```python
from build123d import *

# Parameters (mm, degrees)
ESQUISSE1_W             = 61
ESQUISSE1_H             = 78
BOSS_EXTRU_1_DEPTH      = 2
ESQUISSE2_W             = 61
ESQUISSE2_H             = 78
ESQUISSE2_W_2           = 57
ESQUISSE2_H_2           = 74
BOSS_EXTRU_2_DEPTH      = 7
ESQUISSE3_W             = 59
ESQUISSE3_H             = 76
ESQUISSE3_W_2           = 57
ESQUISSE3_H_2           = 74
BOSS_EXTRU_3_DEPTH      = 4
ESQUISSE4_R             = 2.5
BOSS_EXTRU_4_DEPTH      = 4
ESQUISSE6_W             = 12
ESQUISSE6_H             = 20
ENL_V_MAT_EXTRU_1_DEPTH = 3
ESQUISSE7_W             = 17
ESQUISSE7_H             = 13
ESQUISSE7_W_2           = 9.5
ESQUISSE7_H_2           = 16
ESQUISSE7_W_3           = 7
ENL_V_MAT_EXTRU_2_DEPTH = 3
ESQUISSE5_R             = 1
ENL_V_MAT_EXTRU_3_DEPTH = 4
CHANFREIN1_SIZE         = 3
BOSS_EXTRU_5_DEPTH      = 5
ENL_V_MAT_EXTRU_4_REACH = 7
ESQUISSE9_R             = 2.5
CONG_1_R                = 1
CONG_2_R                = 1
CONG_3_R                = 1


with BuildPart() as part:
    # Esquisse1 → Boss.-Extru.1 (new body)
    with BuildSketch(Plane.XY):
        Rectangle(ESQUISSE1_W, ESQUISSE1_H)
    extrude(amount=BOSS_EXTRU_1_DEPTH)

    # Esquisse2 → Boss.-Extru.2 (add)
    with BuildSketch(Plane.XY.offset(2)):
        Rectangle(ESQUISSE2_W, ESQUISSE2_H)
        Rectangle(ESQUISSE2_W_2, ESQUISSE2_H_2, mode=Mode.SUBTRACT)
    extrude(amount=BOSS_EXTRU_2_DEPTH)

    # Esquisse3 → Boss.-Extru.3 (add)
    with BuildSketch(Plane.XY.offset(9)):
        Rectangle(ESQUISSE3_W, ESQUISSE3_H)
        Rectangle(ESQUISSE3_W_2, ESQUISSE3_H_2, mode=Mode.SUBTRACT)
    extrude(amount=BOSS_EXTRU_3_DEPTH)

    # Esquisse4 → Boss.-Extru.4 (add)
    with BuildSketch(Plane.XY.offset(2)):
        with Locations((-24, 19.6)):
            Circle(ESQUISSE4_R)
        with Locations((24.2, 18.3)):
            Circle(ESQUISSE4_R)
        with Locations((8.9, -32.5)):
            Circle(ESQUISSE4_R)
        with Locations((-19, -32.5)):
            Circle(ESQUISSE4_R)
    extrude(amount=BOSS_EXTRU_4_DEPTH)

    # Esquisse6 → Enlèv. mat.-Extru.1 (cut)
    with BuildSketch(Plane.XZ.offset(39)):
        with Locations((-10, 14.5)):
            Rectangle(ESQUISSE6_W, ESQUISSE6_H)
    extrude(amount=-ENL_V_MAT_EXTRU_1_DEPTH, mode=Mode.SUBTRACT)

    # Esquisse7 → Enlèv. mat.-Extru.2 (cut)
    with BuildSketch(Plane(origin=(0, 39, 0), x_dir=(1, 0, 0), z_dir=(0, 1, 0))):
        with Locations((13.5, -13.5)):
            Rectangle(ESQUISSE7_W, ESQUISSE7_H)
        with Locations((-7.75, -12)):
            Rectangle(ESQUISSE7_W_2, ESQUISSE7_H_2)
        with Locations((-18, -13.5)):
            Rectangle(ESQUISSE7_W_3, ESQUISSE7_H)
    extrude(amount=-ENL_V_MAT_EXTRU_2_DEPTH, mode=Mode.SUBTRACT)

    # Esquisse5 → Enlèv. mat.-Extru.3 (cut)
    with BuildSketch(Plane.XY.offset(6)):
        with Locations((-24, 19.6)):
            Circle(ESQUISSE5_R)
        with Locations((24.2, 18.3)):
            Circle(ESQUISSE5_R)
        with Locations((8.9, -32.5)):
            Circle(ESQUISSE5_R)
        with Locations((-19, -32.5)):
            Circle(ESQUISSE5_R)
    extrude(amount=-ENL_V_MAT_EXTRU_3_DEPTH, mode=Mode.SUBTRACT)

    # Chanfrein1
    chanfrein1_edges = [part.edges().sort_by_distance(p)[0] for p in [
        (-28.5, -37, 7.5),
        (28.5, -37, 7.5),
        (28.5, 37, 7.5),
        (-28.5, 37, 7.5),
    ]]
    chamfer(chanfrein1_edges, length=CHANFREIN1_SIZE)

    # Esquisse8 → Boss.-Extru.5 (add)
    with BuildSketch(Plane(origin=(0, 0, 0), x_dir=(-1, 0, 0), z_dir=(0, 0, -1))):
        with BuildLine():
            Line((-30.5, 5), (-35.5, 5))
            ThreePointArc((-35.5, 5), (-40.5, 0), (-35.5, -5))
            Line((-35.5, -5), (-30.5, -5))
            Line((-30.5, -5), (-30.5, 5))
        make_face()
        with BuildLine():
            Line((30.5, -5), (35.5, -5))
            ThreePointArc((35.5, -5), (40.5, 0), (35.5, 5))
            Line((35.5, 5), (30.5, 5))
            Line((30.5, 5), (30.5, -5))
        make_face()
    extrude(amount=-BOSS_EXTRU_5_DEPTH)

    # Esquisse9 → Enlèv. mat.-Extru.4 (cut, up to next)
    with BuildSketch(Plane.XY.offset(5), mode=Mode.PRIVATE) as enl_v_mat_extru_4_sk1:
        with Locations((-35.5, 0)):
            Circle(ESQUISSE9_R)
    enl_v_mat_extru_4_tool1 = extrude(enl_v_mat_extru_4_sk1.sketch, amount=-ENL_V_MAT_EXTRU_4_REACH, mode=Mode.PRIVATE) & part.part
    add(enl_v_mat_extru_4_tool1.solids().sort_by_distance((-35.5, 0, 5))[0], mode=Mode.SUBTRACT)
    # Esquisse9 → Enlèv. mat.-Extru.4 (cut, up to next)
    with BuildSketch(Plane.XY.offset(5), mode=Mode.PRIVATE) as enl_v_mat_extru_4_sk2:
        with Locations((35.5, 0)):
            Circle(ESQUISSE9_R)
    enl_v_mat_extru_4_tool2 = extrude(enl_v_mat_extru_4_sk2.sketch, amount=-ENL_V_MAT_EXTRU_4_REACH, mode=Mode.PRIVATE) & part.part
    add(enl_v_mat_extru_4_tool2.solids().sort_by_distance((35.5, 0, 5))[0], mode=Mode.SUBTRACT)

    # Congé1
    cong_1_edges = [part.edges().sort_by_distance(p)[0] for p in [
        (-38, 0, 5),
        (33, 0, 5),
    ]]
    fillet(cong_1_edges, radius=CONG_1_R)

    # Congé2
    cong_2_edges = [part.edges().sort_by_distance(p)[0] for p in [
        (30.5, -5, 2.5),
        (30.5, 5, 2.5),
        (30.5, 0, 5),
        (-30.5, 5, 2.5),
        (-30.5, -5, 2.5),
        (-30.5, 0, 5),
    ]]
    fillet(cong_2_edges, radius=CONG_2_R)

    # Congé3
    cong_3_edges = [part.edges().sort_by_distance(p)[0] for p in [
        (0, -37, 2),
        (-28.5, 0, 2),
        (28.5, 0, 2),
        (0, 37, 2),
        (-27, -35.5, 2),
        (-27, 35.5, 2),
        (27, 35.5, 2),
        (27, -35.5, 2),
    ]]
    fillet(cong_3_edges, radius=CONG_3_R)


solid = part.part
```
The model under review builds one solid part; all positions refer to its coordinate system, in mm. A direction names the side the tool comes from. Round coordinates to 2 decimals unless told otherwise and drop trailing zeros. Order: outer loops, then holes, each group sorted by start corner. A loop starts at its lowest first (then second) coordinate and runs counter-clockwise, first axis right, second up.
Item 1: Add section A-A, the plane y = 0. Count the separate pieces of the cut face and the enclosed holes in it, and give its area (3 significant figures).
Working result:
separate pieces: 3
enclosed holes: 0
area: 208 mm2
Item 2: Add section B-B, the plane z = 12. State the section outline as (x, y) points.
Working result:
outline: (-29.5, -38) - (-16, -38) - (-16, -37) - (-25.5, -37) - (-28.5, -34) - (-28.5, 34) - (-25.5, 37) - (-21.5, 37) - (-21.5, 38) - (-29.5, 38) - close; (-14.5, 37) - (-12.5, 37) - (-12.5, 38) - (-14.5, 38) - close; (-4, -38) - (29.5, -38) - (29.5, 38) - (22, 38) - (22, 37) - (25.5, 37) - (28.5, 34) - (28.5, -34) - (25.5, -37) - (-4, -37) - close; (-3, 37) - (5, 37) - (5, 38) - (-3, 38) - close
Item 3: To check wall thickness, follow probe 1 along Y at (x, z) = (24.2, 2.95); probe 2 along X at (y, z) = (-27, 7.25); probe 3 along X at (y, z) = (-28, 10.5). State the ranges of each line that lie inside material, in increasing order.
Working result:
probe 1: y = -39 to -37, 15.8 to 17.3, 19.3 to 20.8, 37 to 39
probe 2: x = -30.5 to -28.5, 28.5 to 30.5
probe 3: x = -29.5 to -28.5, 28.5 to 29.5
Item 4: For pin 1 (2 mm diameter, centred on x = 24, y = 18, fed in from +Z); pin 2 (6 mm diameter, centred on x = 16, y = -15.5, fed in from +Z); pin 3 (0.6 mm diameter, centred on x = -13.5, z = 11.5, fed in from +Y), all flat-tipped, find the tip position at first contact; note any pin that passes through.
Working result:
pin 1: stops at z = 6
pin 2: stops at z = 2
pin 3: stops at y = 38
Item 5: Add section D-D, the plane y = 27.5. State the section outline as (x, z) points.
Working result:
outline: (-30.5, 0) - (30.5, 0) - (30.5, 9) - (29.5, 9) - (29.5, 13) - (28.5, 13) - (28.5, 3) arc R1 cw to (27.5, 2) - (-27.5, 2) arc R1 cw to (-28.5, 3) - (-28.5, 13) - (-29.5, 13) - (-29.5, 9) - (-30.5, 9) - close
Item 6: Draft analysis for pull direction X (two halves, no side actions). For faces 1 (the flat face through (-33, -5, 2)), 2 (the cylindrical face through (-19.13, -31.51, 4.03)), state which applies: released by +X, released by -X, zero draft, split by the parting line, or undercut.
Working result:
face 1: zero draft
face 2: undercut
Item 7: Add section C-C, the plane x = -19. State the section outline as (y, z) points, and give its area (3 significant figures).
Working result:
outline: (-39, 0) - (39, 0) - (39, 7) - (37, 7) - (37, 3) arc R1 cw to (36, 2) - (-30, 2) - (-30, 6) - (-31.5, 6) - (-31.5, 2) - (-33.5, 2) - (-33.5, 6) - (-35, 6) - (-35, 2) - (-36, 2) arc R1 cw to (-37, 3) - (-37, 13) - (-38, 13) - (-38, 9) - (-39, 9) - close
area: 196 mm2
Item 8: Machinability: for faces 3 (the flat face through (13, 38, 7)), 4 (the flat face through (-16, -38, 8)), 5 (the cylindrical face through (-23.54, 18.71, 4.03)), which of the approach directions +Z, -Z, +X, -X, +Y, -Y give a long, thin tool a straight path to every point of the face, cutting with its end or side? Answer none if there is none.
Working result:
face 3: +Z, +Y
face 4: +Z, -Y
face 5: +Z
